Source: CAD feature listing. Evaluate the final solid. Frame: model axes, mm. Face numbers are marked on the shaded views. Round coordinates to 2 decimals unless told otherwise and drop trailing zeros. Order: outer loops, then holes, each group sorted by start corner. A loop starts at its lowest first (then second) coordinate and runs counter-clockwise, first axis right, second up. Notation, with made-up numbers: (74.25, -38) - (123.25, -38) arc R17 ccw to (123.25, -11) - close; hole circle Ø8 at (-8, 78.5). An arc over 180 degrees is marked (long way). Return JSON: item names as keys, results as strings. Group by question number.
1) Ray query, line 1 (Y direction, x = -7.75, z = -0.15); line 2 (Z direction, x = -4.5, y = 12.5). Return the intervals inside material, ascending. Write a range as from..to.
2) Section C-C, the plane x = 12. Return loops of the section in (y, z), plus the area to 3 significant figures.
3) Mould query, pull axis X, two halves, no side actions, for the marked faces 1, 2, 3 and 4. Classes: pulls with the +X half, pulls with the -X half, needs draft (parallel to the pull), parting line crosses it, or undercut.
4) Section A-A, the plane x = 6.5. Return loops of the section in (y, z) (3 decimals).
5) Section B-B, the plane y = -3.75. Return loops of the section in (x, z).
6) Contact query for flat-ended pins moving along their axis: P1, Ø3, axis at x = 7.5, y = 3.5, coming from the +Z side; P2, Ø1.2, axis at y = -5.5, z = 0, coming from the -X side; P3, Ø2, axis at y = -5.76, z = 0.71, coming from the +X side; P4, Ø1, axis at y = 5, z = 1, coming from the +X side. Output: stop coordinate, or through.
```python
from build123d import *

# Parameters (mm, degrees)
F0_W      = 25.4
F0_H      = 25.4
F1_DEPTH  = 2.54
F2_W      = 10.16
F2_H      = 2.54
F3_DEPTH  = 1.4224
F5_W      = 1.143
F5_H      = 1.4224
F5_W_2    = 3.81
F6_DEPTH  = 25.4
F7_DEPTH  = 25.4
F8_W      = 8.763
F8_H      = 2.54
F9_DEPTH  = 0.889
F10_W     = 22.86
F10_H     = 0.0508
F11_DEPTH = 25.4


with BuildPart() as f1:
    # F0 (on Top) → F1 (new body)
    with BuildSketch(Plane.XY):
        with Locations((2.984056, 5.665214)):
            Rectangle(F0_W, F0_H)
    extrude(amount=-F1_DEPTH)

    # F2 (on face) → F3 (join)
    with BuildSketch(Plane.XY):
        with Locations((2.984056, -5.764786)):
            Rectangle(F2_W, F2_H)
    extrude(amount=F3_DEPTH)

    # F5 (on face) → F6 (cut)
    with BuildSketch(Plane.XZ.offset(7.034786)):
        with Locations((-1.524444, 0.7112)):
            Rectangle(F5_W, F5_H)
        with Locations((2.984056, 0.7112)):
            Rectangle(F5_W_2, F5_H)
        with Locations((7.492556, 0.7112)):
            Rectangle(F5_W, F5_H)
    extrude(amount=-F6_DEPTH, mode=Mode.SUBTRACT)

    # F4 (on face) → F7 (cut)
    with BuildSketch(Plane(origin=(-2.095944, 0, 0), x_dir=(0, -1, 0), z_dir=(-1, 0, 0))):
        Polygon((4.494786, 0), (5.224647, 1.4224), (4.494786, 1.4224), align=None)
        with BuildLine():
            ThreePointArc((5.224647, 1.091172), (5.565511, 0.081583), (6.425186, 0.7112))
            ThreePointArc((6.425186, 0.7112), (6.39704, 0.901944), (6.315001, 1.076428))
            ThreePointArc((6.315001, 1.076428), (5.773715, 1.37154), (5.224647, 1.091172))
        make_face()
        with BuildLine():
            ThreePointArc((5.224647, 1.091172), (5.773715, 1.37154), (6.315001, 1.076428))
            Line((6.315001, 1.076428), (6.315001, 1.4224))
            Line((6.315001, 1.4224), (5.224647, 1.4224))
            Line((5.224647, 1.4224), (5.224647, 1.091172))
        make_face()
        Polygon((7.034786, 1.4224), (6.315001, 1.4224), (7.034786, 0), align=None)
    extrude(amount=-F7_DEPTH, mode=Mode.SUBTRACT)

    # F8 (on face) → F9 (cut)
    with BuildSketch(Plane.XY):
        with Locations((11.302556, -5.764786)):
            Rectangle(F8_W, F8_H)
        with Locations((-5.334444, -5.764786)):
            Rectangle(F8_W, F8_H)
    extrude(amount=-F9_DEPTH, mode=Mode.SUBTRACT)

    # F10 (on face) → F11 (cut)
    with BuildSketch(Plane.YZ.offset(15.684056)):
        with Locations((6.935214, -0.0254)):
            Rectangle(F10_W, F10_H)
    extrude(amount=-F11_DEPTH, mode=Mode.SUBTRACT)


solid = f1.part
```
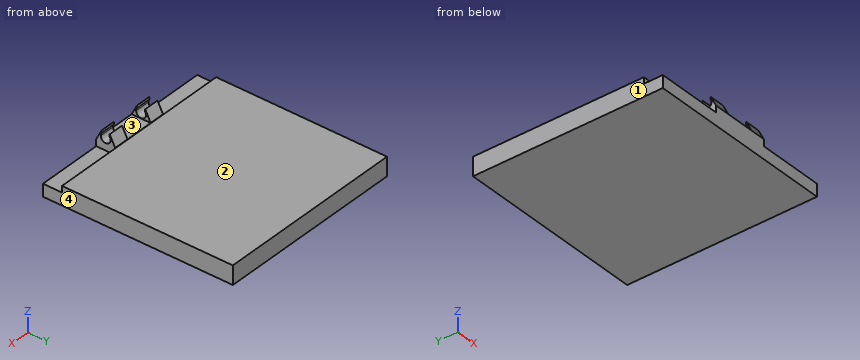
Geometry check:
{
 "1": {"line 1": "-4.49..18.37", "line 2": "-2.54..-0.05"},
 "2": {"outline": "(-7.03, -2.54) - (18.37, -2.54) - (18.37, -0.05) - (-4.49, -0.05) - (-4.49, -0.89) - (-7.03, -0.89) - close", "area": "61.1 mm2"},
 "3": {"face 1": "pulls with the -X half", "face 2": "needs draft", "face 3": "undercut", "face 4": "pulls with the +X half"},
 "4": {"outline": "(-7.035, -2.54) - (18.365, -2.54) - (18.365, -0.051) - (-4.495, -0.051) - (-4.495, 0) - (-5.225, 1.422) - (-5.225, 1.091) arc R0.66 cw (long way) to (-6.425, 0.711) arc R0.66 cw to (-6.315, 1.076) - (-6.315, 1.422) - (-7.035, 0) - close"},
 "5": {"outline": "(-9.72, -2.54) - (15.68, -2.54) - (15.68, -0.05) - (-9.72, -0.05) - close"},
 "6": {"P1": "z = -0.05", "P2": "x = -0.95", "P3": "x = 6.92", "P4": "through"}
}
